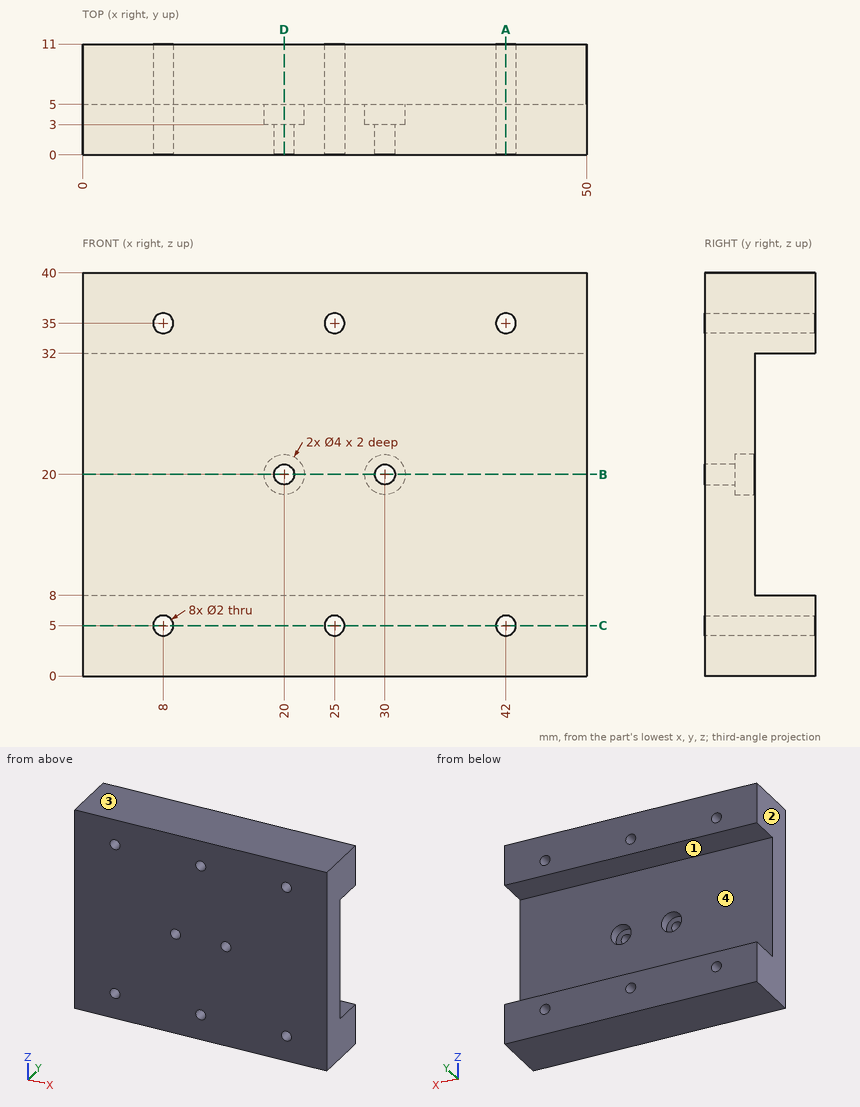
Print and shaded views of the part. All mm, measured from the part's lowest x, y and z. Round coordinates to 2 decimals unless told otherwise and drop trailing zeros. Write each loop counter-clockwise with the first axis right and the second up, starting at its lowest first coordinate (ties: lowest second). Pieces come first, ordered by that corner, then holes. Notation, with made-up numbers: M 32,-19.75 L 69,-19.75 A20 ccw 69,10.25 Z; hole C -17.5,21 d5. An arc over 180 degrees is marked long. One line per question, with ' | ' between items.
(1) Probe line 1 along Z through (x, y) = (25, 8.5); line 2 along X through (y, z) = (4.5, 20); line 3 along X through (y, z) = (6, 35). List the from-to ranges inside material, lowest first.
Answer key:
line 1: z = 0 to 4, 6 to 8, 32 to 34, 36 to 40 | line 2: x = 0 to 18, 22 to 28, 32 to 50 | line 3: x = 0 to 7, 9 to 24, 26 to 41, 43 to 50
(2) Saw through at A-A on x = 42. Write the cut outline in (y, z).
Answer key:
outline: M 0,0 L 11,0 L 11,4 L 0,4 Z; M 0,6 L 11,6 L 11,8 L 5,8 L 5,32 L 11,32 L 11,34 L 0,34 Z; M 0,36 L 11,36 L 11,40 L 0,40 Z
(3) Pin check, flat tips, straight feed: pin 1 (2 mm diameter, centred on x = 29.5, z = 20.5, fed in from +Y); pin 2 (3 mm diameter, centred on x = 19, z = 13, fed in from +Y); pin 3 (1.8 mm diameter, centred on x = 42, z = 5, fed in from -Y). Stop position of each tip, or through.
Answer key:
pin 1: stops at y = 3 | pin 2: stops at y = 5 | pin 3: passes through
(4) Saw through at B-B on z = 20. Write the cut outline in (x, y).
Answer key:
outline: M 0,0 L 19,0 L 19,3 L 18,3 L 18,5 L 0,5 Z; M 21,0 L 29,0 L 29,3 L 28,3 L 28,5 L 22,5 L 22,3 L 21,3 Z; M 31,0 L 50,0 L 50,5 L 32,5 L 32,3 L 31,3 Z
(5) Saw through at C-C on z = 5. Write the cut outline in (x, y).
Answer key:
outline: M 0,0 L 7,0 L 7,11 L 0,11 Z; M 9,0 L 24,0 L 24,11 L 9,11 Z; M 26,0 L 41,0 L 41,11 L 26,11 Z; M 43,0 L 50,0 L 50,11 L 43,11 Z
(6) Saw through at D-D on x = 20. Write the cut outline in (y, z).
Answer key:
outline: M 0,0 L 11,0 L 11,8 L 5,8 L 5,18 L 3,18 L 3,19 L 0,19 Z; M 0,21 L 3,21 L 3,22 L 5,22 L 5,32 L 11,32 L 11,40 L 0,40 Z
(7) Two-plate mould, pull along Z, no slides. Class the marked faces 1, 2, 3 and 4: released by +Z, released by -Z, zero draft, split by the parting line, or undercut.
Answer key:
face 1: undercut | face 2: zero draft | face 3: released by +Z | face 4: undercut
